Geometry: final body of the model. Coordinates: model frame, mm. Face numbers are marked on the shaded views. A direction names the side the tool comes from. Give positions to 0.01 mm unless a question says otherwise; leave off trailing zeros. Write each loop counter-clockwise with the first axis right and the second up, starting at its lowest first coordinate (ties: lowest second). Pieces come first, ordered by that corner, then holes.
Q1. Line query: line 1 (Z direction, x = -55, y = 29); line 2 (Z direction, x = 46, y = -33.5); line 3 (Y direction, x = -28.5, z = 50). Output: solid intervals per line, ascending.
Q2. Section C-C (y = -3). Return the cut outline in (x, z).
Q3. Section D-D (z = 34.5). Return the cut outline in (x, y), plus the area to 3 significant figures.
Q4. Section A-A (x = -55). Return the cut outline in (y, z), plus the area to 3 significant figures.
Q5. Pin query (flat end, axial travel): pin 1 Ø6 at (x, y) = (-51, -13.5) entering from -Z; pin 2 Ø24 at (x, y) = (54.5, -6) entering from +Z; pin 3 Ø9 at (y, z) = (-11.5, 41.5) entering from +X. Return the tip coordinate at first contact, or that it passes through.
Q6. Reachability of the marked faces 1, 2, 3 and 4 from +Z, -Z, +X, -X, +Y, -Y: full face, straight path, thin tool, end or side. Return the list, or none.
Q7. Section B-B (z = 13). Return the cut outline in (x, y).
Q8. Mould query, pull axis X, two halves, no side actions, for the marked faces 5, 6 and 7. Classes: +X half, -X half, draft (parallel to the pull), parting line (faces both ways), or undercut.
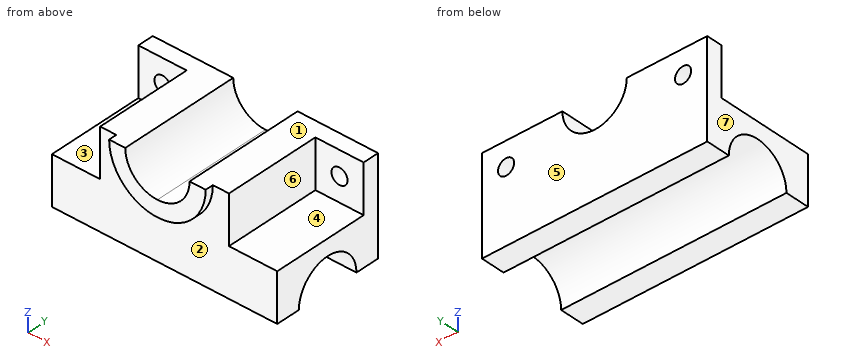
from build123d import *

# Parameters (mm, degrees)
F1_DEPTH = 35
F2_W     = 30
F2_H     = 30
F3_DEPTH = 60
F4_R     = 5
F5_DEPTH = 10.001
F7_DEPTH = 70.001
F8_DEPTH = 40


with BuildPart() as f1:
    # F0 (on Front) → F1 (new body, symmetric)
    with BuildSketch(Plane.XZ):
        with BuildLine():
            Line((0, 30), (0, 0))
            Line((0, 0), (70, 0))
            Line((70, 0), (70, 60))
            Line((70, 60), (30, 60))
            ThreePointArc((30, 60), (21.2132034356, 38.7867965644), (0, 30))
        make_face()
        with BuildLine():
            Line((0, 40), (0, 30))
            ThreePointArc((0, 30), (21.2132034356, 38.7867965644), (30, 60))
            Line((30, 60), (20, 60))
            ThreePointArc((20, 60), (14.1421356237, 45.8578643763), (0, 40))
        make_face()
    extrude(amount=F1_DEPTH, both=True)

    # F2 (on face) → F3 (cut)
    with BuildSketch(Plane.XZ.offset(35)):
        with Locations((55, 45)):
            Rectangle(F2_W, F2_H)
    extrude(amount=-F3_DEPTH, mode=Mode.SUBTRACT)

    # F4 (on face) → F5 (cut, through all)
    with BuildSketch(Plane.XZ.offset(-25)):
        with Locations((55, 45)):
            Circle(F4_R)
    extrude(amount=-F5_DEPTH, mode=Mode.SUBTRACT)

    # F6 (on face) → F7 (cut, through all)
    with BuildSketch(Plane.YZ.offset(70)):
        with BuildLine():
            Line((-20, 0), (20, 0))
            ThreePointArc((20, 0), (0, 20), (-20, 0))
        make_face()
    extrude(amount=-F7_DEPTH, mode=Mode.SUBTRACT)

    # F0 (on Front) → F8 (join)
    with BuildSketch(Plane.XZ):
        with BuildLine():
            Line((0, 40), (0, 30))
            ThreePointArc((0, 30), (21.2132034356, 38.7867965644), (30, 60))
            Line((30, 60), (20, 60))
            ThreePointArc((20, 60), (14.1421356237, 45.8578643763), (0, 40))
        make_face()
    extrude(amount=F8_DEPTH)

    # F9: F1 across plane


with BuildPart() as f1_1:
    add(f1.part)
    add(f1.part.mirror(Plane.YZ))


solid = f1_1.part
Computed:
1. line 1: z = 0 to 40, 50 to 60
1. line 2: z = 0 to 30
1. line 3: y = -35 to 35
2. outline: (-70, 19.77) - (70, 19.77) - (70, 30) - (40, 30) - (40, 60) - (20, 60) arc R20 cw to (-20, 60) - (-40, 60) - (-40, 30) - (-70, 30) - close
3. outline: (-70, 25) - (-40, 25) - (-40, -35) - (-15.8, -35) - (-15.8, -40) - (15.8, -40) - (15.8, -35) - (40, -35) - (40, 25) - (70, 25) - (70, 35) - (-70, 35) - close
3. area: 6,360 mm2
4. outline: (-35, 0) - (-20, 0) arc R20 cw to (20, 0) - (35, 0) - (35, 40) - (25, 40) - (25, 30) - (-35, 30) - close; (25, 50) - (35, 50) - (35, 60) - (25, 60) - close
4. area: 1,670 mm2
5. pin 1: stops at z = 11.3
5. pin 2: stops at z = 30
5. pin 3: stops at x = 40
6. face 1: +Z, +X, -X, +Y, -Y
6. face 2: -Z, -Y
6. face 3: +Z, -X, -Y
6. face 4: +Z, +X, -Y
7. outline: (-70, -35) - (70, -35) - (70, -15.2) - (-70, -15.2) - close; (-70, 15.2) - (70, 15.2) - (70, 35) - (-70, 35) - close
8. face 5: draft
8. face 6: +X half
8. face 7: -X half
